Source: three-view drawing plus pictorial views. Frame: mm from the lowest corner of the part. Give positions to 0.01 mm unless a question says otherwise; leave off trailing zeros. Loops run counter-clockwise (first coordinate to the right, second up) from the corner with the lowest first, then second, coordinate; pieces in that order, holes last.
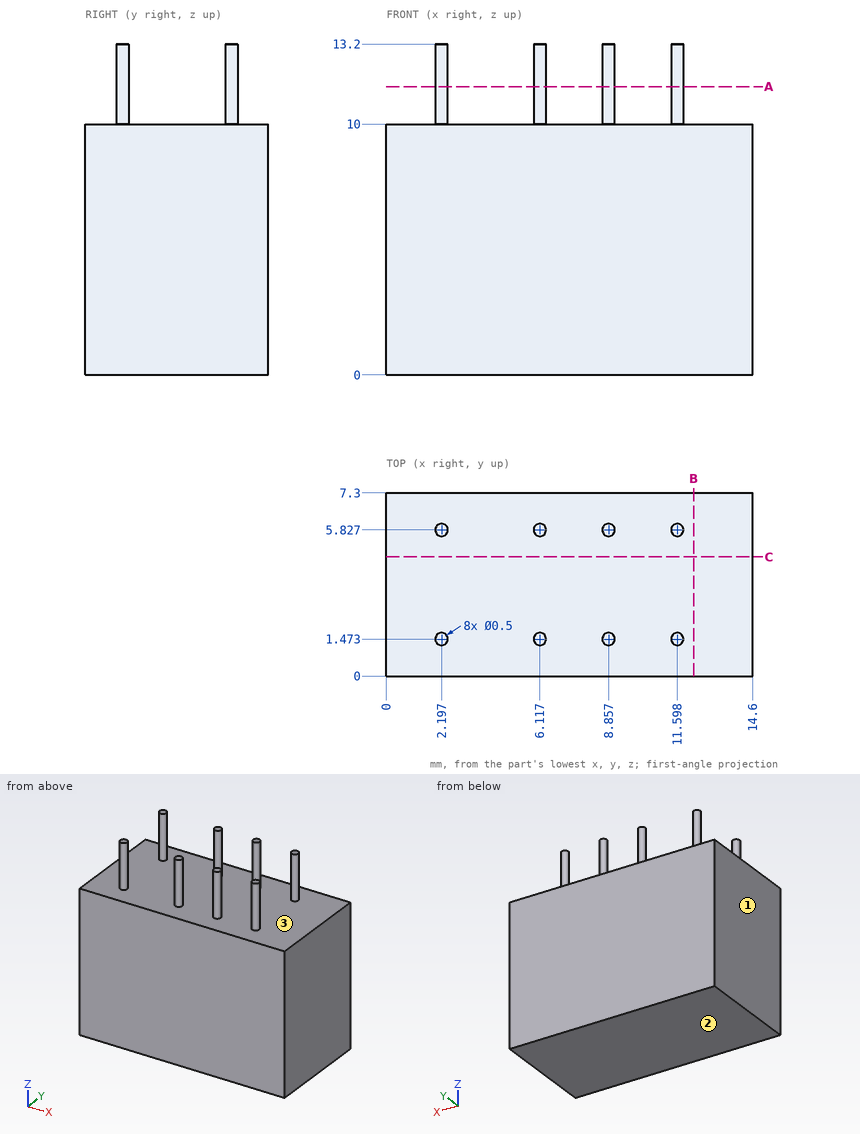
(1) Cut plane B-B (x = 12.25). Return the cut outline in (y, z).
Values follow:
outline: (0, 0) - (7.3, 0) - (7.3, 10) - (0, 10) - close
(2) Ray query, probe 1 along Z at (x, y) = (9, 1.75). Return the intervals inside material, ascending.
Values follow:
probe 1: z = 0 to 10
(3) Pin query (flat end, axial travel): pin 1 Ø1.5 at (x, y) = (4, 5.5) entering from +Z. Return the tip coordinate at first contact, or that it passes through.
Values follow:
pin 1: stops at z = 10
(4) Cut plane C-C (y = 4.75). Return the cut outline in (x, z), and give its area (3 significant figures).
Values follow:
outline: (0, 0) - (14.6, 0) - (14.6, 10) - (0, 10) - close
area: 146 mm2
(5) Cut plane A-A (z = 11.5). Return the cut outline in (x, y).
Values follow:
outline: circle Ø0.5 at (2.2, 1.47); circle Ø0.5 at (2.2, 5.83); circle Ø0.5 at (6.12, 1.47); circle Ø0.5 at (6.12, 5.83); circle Ø0.5 at (8.86, 1.47); circle Ø0.5 at (8.86, 5.83); circle Ø0.5 at (11.6, 1.47); circle Ø0.5 at (11.6, 5.83)
(6) Mould query, pull axis Z, two halves, no side actions, for the marked faces 1, 2 and 3. Classes: +Z half, -Z half, draft (parallel to the pull), parting line (faces both ways), or undercut.
Values follow:
face 1: draft
face 2: -Z half
face 3: +Z half
